Autodesk Inventor part; units mm, degrees
ref_plane "YZ Plane" through (0, 0, 0) normal (1, 0, 0) x (0, 1, 0)
ref_plane "XZ Plane" through (0, 0, 0) normal (0, 1, 0) x (-1, 0, 0)
ref_plane "XY Plane" through (0, 0, 0) normal (0, 0, 1) x (1, 0, 0)
sketch "Szkic1" plane through (0, 0, 0) normal (0, 1, 0) x (-1, 0, 0)
  line L0 (0, 15) -> (0, -15) construction
  line L1 (-4, 15) -> (-4, -15)
  line L2 (4, -15) -> (4, 15)
  arc A0 (4, 15) -> (-4, 15) centre (0, 15) ccw
  arc A1 (-4, -15) -> (4, -15) centre (0, -15) ccw
  circle A2 centre (0, -15) radius 2.5
  circle A3 centre (0, 15) radius 2.5
  line L3 (0, 15) -> (0, 5)
  line L4 (0, 5) -> (4, 5)
  line L5 (0, 5) -> (-4, 5)
  point P0 (0, 0)
  dimension "d0" = 15
  dimension "d1" = 8
  dimension "d2" = 5
  dimension "d3" = 5
  dimension "d6" = 10
extrude "Wyciągnięcie proste1" add sketch "Szkic1" along normal mid plane 10 contours A0 L2 L4 L5 L1 | L5 L4 L2 A1 L1 | A2 | A3
extrude "Wyciągnięcie proste2" cut sketch "Szkic1" along normal mid plane 4 contours A0 L2 L4 L5 L1
extrude "Wyciągnięcie proste3" cut sketch "Szkic1" along normal mid plane 14.5 contours A3
mirror "Odbij1" about plane through (0, 0, 0) normal (0, 0, 1) of "Wyciągnięcie proste2", "Wyciągnięcie proste3"
fillet "Zaokrąglenie1" radius 2 4 edges at (-4, 0, 5) (-4, 0, -5) (4, 0, -5) (4, 0, 5)
sketch "Szkic2" plane through (0, 5, 0) normal (0, 1, 0) x (1, 0, 0)
  circle A0 centre (0, 15) radius 2.5
  circle A1 centre (0, 15) radius 4
  circle A2 centre (0, 15) radius 2.5
  point P0 (0, 0)
extrude "Wyciągnięcie proste4" add sketch "Szkic2" against normal up to surface (10 mm away)
properties part number "connector"
Check sheet for the modelled part. Datum: model origin and axes. Units: mm. A direction names the side the tool comes from. Give positions to 0.01 mm unless a question says otherwise; leave off trailing zeros. Order: outer loops, then holes, each group sorted by start corner. A loop starts at its lowest first (then second) coordinate and runs counter-clockwise, first axis right, second up. Notation, with made-up numbers: M -26.75,80 L -0.75,80 A12 ccw -0.75,88 Z; hole C -2.5,9.25 d2. An arc over 180 degrees is marked long. Answer as CSV lines item,"result". Start each with the question number.
Item 1: Cross-section at B-B on y = -0.75. Enter the section's corners in (x, z), plus the area to 3 significant figures.
Item 2: Thickness scan on line 1 (Z direction, x = 0, y = 3.2); line 2 (Z direction, x = 0, y = 0.6); line 3 (Y direction, x = 2.5, z = 11.5). Record the ranges inside material, lowest first. Write a range as [from, to].
Item 3: Cross-section at A-A on x = 0. Enter the section's corners in (y, z).
Item 4: Mould release check, pull along X, two halves, no side actions. Record for faces 4 (the face through (0.54, -3.48, 12.56)), 5 (the face through (0, -4, 19)), 6 (the face through (0, 2, 11)): +X half, -X half, draft (parallel to the pull), parting line (faces both ways), or undercut.
Item 5: Tool access check on faces 1 (the face through (0, 0, -5)), 2 (the face through (-0.867, -0.07, -18.905)), 3 (the face through (3.4, 0.03, 4.43)). Record the directions out of +Z, -Z, +X, -X, +Y, -Y that give a thin tool (end or side, any length) a straight path to the whole face; none if there is none.
Item 6: Cross-section at C-C on z = 9. Enter the section's corners in (x, y), plus the area to 3 significant figures.
Item 7: Cross-section at D-D on y = 3.5. Enter the section's corners in (x, z).
Item 8: Gauge pin test, flat ends, axial feed: P1, Ø1, axis at x = 1.5, y = 3.5, coming from the +Z side; P2, Ø3, axis at x = 0, z = 15, coming from the +Y side; P3, Ø1.5, axis at x = -2, y = -4, coming from the -Z side. Record the tip position at first contact, or that the pin passes through.
Established:
1,outline,"C 0,-15 d8; M -4,-3 A2 ccw -2,-5 L 2,-5 A2 ccw 4,-3 L 4,3 A2 ccw 2,5 L -2,5 A2 ccw -4,3 Z; hole C 0,-15 d5"
1,area,"107 mm^2"
2,line 1,"z = [-19, -17.5], [-12.5, 12.5], [17.5, 19]"
2,line 2,"z = [-19, -17.5], [-12.5, -11], [-5, 5]"
2,line 3,"y = [-5, -2], [2, 5]"
3,outline,"M -5,-19 L 5,-19 L 5,-17.5 L -5,-17.5 Z; M -5,-12.5 L 5,-12.5 L 5,12.5 L 2,12.5 L 2,5 L -2,5 L -2,12.5 L -5,12.5 Z; M -5,17.5 L -2,17.5 L -2,19 L -5,19 Z; M 2,17.5 L 5,17.5 L 5,19 L 2,19 Z; hole M -2,-11 L 2,-11 L 2,-5 L -2,-5 Z"
4,face 4,"undercut"
4,face 5,"parting line"
4,face 6,"draft"
5,face 1,"+X, -X"
5,face 2,"none"
5,face 3,"+Z, +X"
6,outline,"M -4,-5 L 4,-5 L 4,-2 L -4,-2 Z; M -4,2 L 4,2 L 4,5 L -4,5 Z"
6,area,"48.0 mm^2"
7,outline,"M -4,-15 A4 ccw 4,-15 L 4,15 A4 ccw -4,15 Z; hole C 0,-15 d5; hole C 0,15 d5"
8,P1,"stops at z = 18.87"
8,P2,"passes through"
8,P3,"stops at z = -18.8"
